Source: three-view drawing plus pictorial views. Frame: mm from the lowest corner of the part. A direction names the side the tool comes from. Coordinates: 2 decimals unless noted, no trailing zeros. Order: outer loops, then holes, each group sorted by start corner. A loop starts at its lowest first (then second) coordinate and runs counter-clockwise, first axis right, second up. Notation, with made-up numbers: (41.5, -25.5) -> (81.5, -25.5) arc R11 cw to (81.5, -5.5) -> close; hole circle Ø2 at (31, 64). An arc over 180 degrees is marked (long way). Use CSV: the item, a comma, the result in double quotes. Start each with the question number.
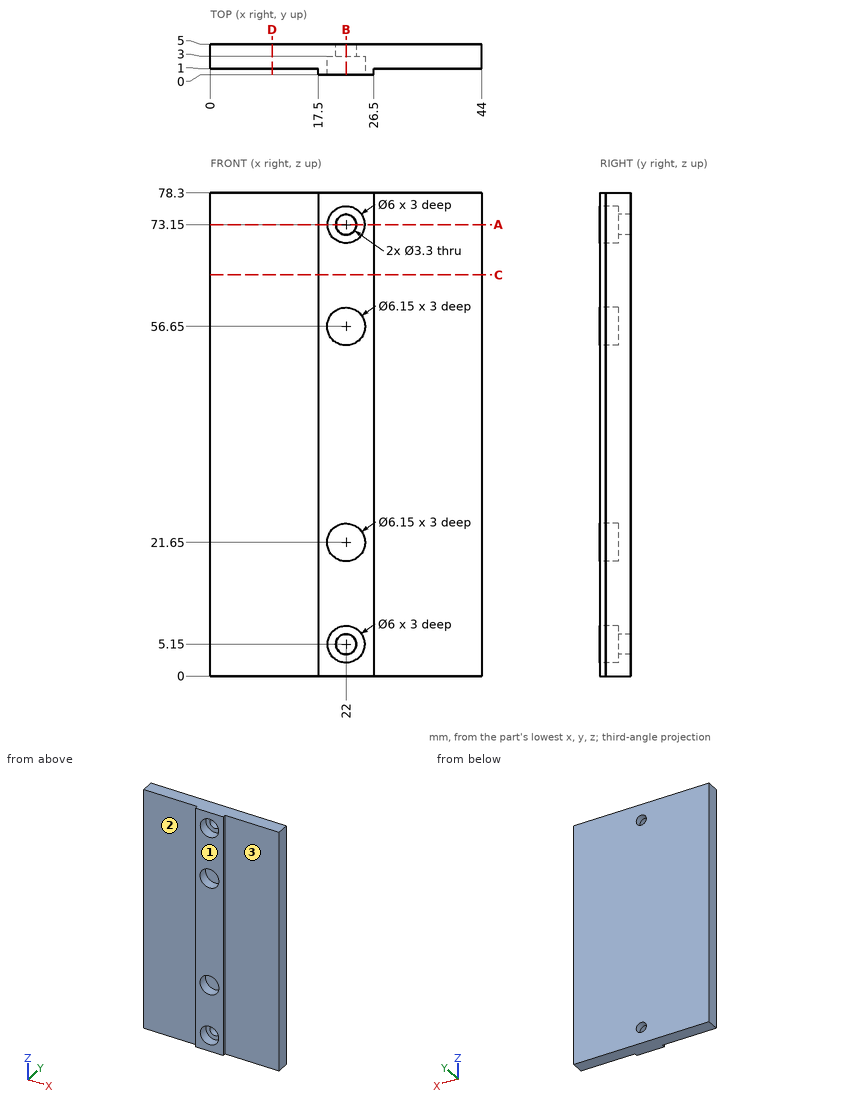
1. Section C-C on z = 65. Return loops of the section in (x, y), then the cut area to 3 significant figures.
2. Contact query for flat-ended pins moving along their axis: P1, Ø5, axis at x = 22, z = 56.65, coming from the -Y side; P2, Ø2.5, axis at x = 22, z = 73.15, coming from the -Y side; P3, Ø0.5, axis at y = 0.5, z = 39.5, coming from the +X side. Output: stop coordinate, or through.
3. Section A-A on z = 73.15. Return loops of the section in (x, y).
4. Section B-B on x = 22. Return loops of the section in (y, z) (3 decimals), then the cut area to 3 significant figures.
5. Material intervals for line 1 along Z through (x, y) = (22, 1.15) (3 decimals); line 2 along Z through (x, y) = (20, 2.2); line 3 along X through (y, z) = (3.7, 5.15), sorted ascending.
6. Section D-D on x = 10. Return loops of the section in (y, z), then the cut area to 3 significant figures.
7. Access query for the marked faces 1, 2 and 3. Directions: +Z, -Z, +X, -X, +Y, -Y. A direction counts if a zero-diameter tool reaches every point of the face in a straight line with its end or side. Return the directions, or none.
Values follow:
1,outline,"(0, 1) -> (17.5, 1) -> (17.5, 0) -> (26.5, 0) -> (26.5, 1) -> (44, 1) -> (44, 5) -> (0, 5) -> close"
1,area,"185 mm2"
2,P1,"stops at y = 3"
2,P2,"passes through"
2,P3,"stops at x = 26.5"
3,outline,"(0, 1) -> (17.5, 1) -> (17.5, 0) -> (19, 0) -> (19, 3) -> (20.35, 3) -> (20.35, 5) -> (0, 5) -> close; (23.65, 3) -> (25, 3) -> (25, 0) -> (26.5, 0) -> (26.5, 1) -> (44, 1) -> (44, 5) -> (23.65, 5) -> close"
4,outline,"(0, 0) -> (5, 0) -> (5, 3.5) -> (3, 3.5) -> (3, 2.15) -> (0, 2.15) -> close; (0, 8.15) -> (3, 8.15) -> (3, 6.8) -> (5, 6.8) -> (5, 71.5) -> (3, 71.5) -> (3, 70.15) -> (0, 70.15) -> (0, 59.725) -> (3, 59.725) -> (3, 53.575) -> (0, 53.575) -> (0, 24.725) -> (3, 24.725) -> (3, 18.575) -> (0, 18.575) -> close; (0, 76.15) -> (3, 76.15) -> (3, 74.8) -> (5, 74.8) -> (5, 78.3) -> (0, 78.3) -> close"
4,area,"305 mm2"
5,line 1,"z = 0 to 2.15, 8.15 to 18.575, 24.725 to 53.575, 59.725 to 70.15, 76.15 to 78.3"
5,line 2,"z = 0 to 2.91, 7.39 to 19.31, 23.99 to 54.31, 58.99 to 70.91, 75.39 to 78.3"
5,line 3,"x = 0 to 20.35, 23.65 to 44"
6,outline,"(1, 0) -> (5, 0) -> (5, 78.3) -> (1, 78.3) -> close"
6,area,"313 mm2"
7,face 1,"+Z, -Z, +X, -X, -Y"
7,face 2,"+Z, -Z, -X, -Y"
7,face 3,"+Z, -Z, +X, -Y"
